```python
from build123d import *

# Parameters (mm, degrees)
F0_W      = 50
F0_H      = 70
F1_DEPTH  = 95
F1_FACE_W = 70
F1_FACE_H = 95
F2_DEPTH  = 60.59026
F3_R      = 32.333924
F4_DEPTH  = 25
F5_R      = 16.327399
F6_DEPTH  = 10


with BuildPart() as f1:
    # F0 (on Top) → F1 (new body)
    with BuildSketch(Plane.XY):
        with Locations((25, 35)):
            Rectangle(F0_W, F0_H)
    extrude(amount=F1_DEPTH)

    # F1_face (on face) → F2 (join)
    with BuildSketch(Plane(origin=(50, 35, 47.5), x_dir=(0, 1, 0), z_dir=(1, 0, 0))):
        Rectangle(F1_FACE_W, F1_FACE_H)
    extrude(amount=F2_DEPTH)

    # F3 (on face) → F4 (join)
    with BuildSketch(Plane.YZ.offset(110.59026)):
        with Locations((46.391159, 41.153282)):
            Circle(F3_R)
    extrude(amount=F4_DEPTH)

    # F5 (on face) → F6 (join)
    with BuildSketch(Plane.YZ.offset(135.59026)):
        with Locations((46.391159, 41.153282)):
            Circle(F5_R)
    extrude(amount=-F6_DEPTH)


solid = f1.part
```
The listing builds one solid part. Answer for the finished solid, in the listing's coordinates (mm). A direction names the side the tool comes from. Give positions to 0.01 mm unless a question says otherwise; leave off trailing zeros. Write each loop counter-clockwise with the first axis right and the second up, starting at its lowest first coordinate (ties: lowest second). Pieces come first, ordered by that corner, then holes. Notation, with made-up numbers: (74, 27) -> (112, 27) arc R19 ccw to (112, 38) -> close; hole circle Ø9 at (26, 40). An arc over 180 degrees is marked (long way). Write item = value, one per line. Start each with the question number.
1) The part is cut by section C-C, the plane x = 83.5. Determine the outline of the cut face in (y, z), and give its area (3 significant figures).
2) The part is cut by section B-B, the plane y = 25.5. Determine the outline of the cut face in (x, z).
3) Which of the six approach directions +Z, -Z, +X, -X, +Y, -Y give full straight-line access (tool end or side, diameter ignored) to faces 1 (the face through (55, 70, 47)), 2 (the face through (122.915, 61.311, 12.468)), 3 (the face through (55, 0, 47))?
4) The part is cut by section A-A, the plane z = 39. Determine the outline of the cut face in (x, y).
5) Straight lines are drawn through the part: line 1 along Y through (x, z) = (108.5, 31); line 2 along X through (y, z) = (6.5, 40.5); line 3 along Z through (x, y) = (112, 22.5). For each, find the intervals that lie inside material, in ascending order.
6) The part is cut by section D-D, the plane z = 84.5. Determine the outline of the cut face in (x, y).
7) Each of these flat-tipped pins is pushed along its axis until it touches: pin 1 (1.5 mm diameter, centred on x = 114, y = 60.5, fed in from +Z); pin 2 (2 mm diameter, centred on x = 84.5, z = 18.5, fed in from +Y); pin 3 (4.5 mm diameter, centred on y = 73.5, z = 46.5, fed in from -X). Where does it stop, or does it pass through?
Solutions:
q1.outline = (0, 0) -> (70, 0) -> (70, 95) -> (0, 95) -> close
q1.area = 6,650 mm²
q2.outline = (0, 0) -> (110.59, 0) -> (110.59, 16.47) -> (135.59, 16.47) -> (135.59, 65.83) -> (110.59, 65.83) -> (110.59, 95) -> (0, 95) -> close
q3.face_1 = +Z, -Z, -X, +Y
q3.face_2 = +X
q3.face_3 = +Z, -Z, +X, -X, -Y
q4.outline = (0, 0) -> (110.59, 0) -> (110.59, 14.13) -> (135.59, 14.13) -> (135.59, 78.65) -> (110.59, 78.65) -> (110.59, 70) -> (0, 70) -> close
q5.line_1 = 0 to 70
q5.line_2 = 0 to 110.59
q5.line_3 = 19.37 to 62.94
q6.outline = (0, 0) -> (110.59, 0) -> (110.59, 70) -> (0, 70) -> close
q7.pin_1 = 70.6
q7.pin_2 = 70
q7.pin_3 = 110.59
